Read the model definition and answer for the solid it produces. Units are mm, in the model's axes. Face numbers are marked on the shaded views. Round coordinates to 2 decimals unless told otherwise and drop trailing zeros. Write each loop counter-clockwise with the first axis right and the second up, starting at its lowest first coordinate (ties: lowest second). Pieces come first, ordered by that corner, then holes. Notation, with made-up numbers: (33.5, 85.5) -> (71.5, 85.5) arc R30 ccw to (71.5, 123.5) -> close; hole circle Ø3 at (-27.5, -33). An arc over 180 degrees is marked (long way). Return JSON: item names as keys, results as strings.
from build123d import *

# Parameters (mm, degrees)
SKETCH2_R           = 28.194
SKETCH2_R_2         = 25.654
BOSS_EXTRUDE1_DEPTH = 76.2
SKETCH3_R           = 9.652
CUT_EXTRUDE1_DEPTH  = 76.2
CIRPATTERN1_COUNT   = 2
CIRPATTERN1_ANGLE   = 60
CIRPATTERN2_COUNT   = 2
CIRPATTERN3_COUNT   = 2
CIRPATTERN3_ANGLE   = 120


with BuildPart() as part:
    # Sketch2 → Boss-Extrude1 (new body)
    with BuildSketch(Plane(origin=(0, 0, 0), x_dir=(1, 0, 0), z_dir=(0, 1, 0))):
        with Locations(Location((0, 0, 0), (0, 0, 90))):
            Circle(SKETCH2_R)
        with Locations(Location((0, 0, 0), (0, 0, 90))):
            Circle(SKETCH2_R_2, mode=Mode.SUBTRACT)
    extrude(amount=BOSS_EXTRUDE1_DEPTH)

    # Sketch3 → Cut-Extrude1 (cut)
    with BuildSketch(Plane.XY):
        with Locations(Location((0, 38.1, 0), (0, 0, 90))):
            Circle(SKETCH3_R)
    cut_extrude1 = extrude(amount=-CUT_EXTRUDE1_DEPTH, mode=Mode.SUBTRACT)

    # CirPattern1: Cut-Extrude1 ×2 about axis
    cirpattern1_axis = Axis((0, 76.2, 0), (0, -1, 0))
    for i in range(1, CIRPATTERN1_COUNT):
        add(cut_extrude1.rotate(cirpattern1_axis, i * CIRPATTERN1_ANGLE / (CIRPATTERN1_COUNT - 1)), mode=Mode.SUBTRACT)

    # CirPattern2: Cut-Extrude1 ×2 about axis
    cirpattern2_axis = Axis((0, 76.2, 0), (0, -1, 0))
    for i in range(1, CIRPATTERN2_COUNT):
        add(cut_extrude1.rotate(cirpattern2_axis, i * 360 / CIRPATTERN2_COUNT), mode=Mode.SUBTRACT)

    # CirPattern3: Cut-Extrude1 ×2 about axis
    cirpattern3_axis = Axis((0, 76.2, 0), (0, 1, 0))
    for i in range(1, CIRPATTERN3_COUNT):
        add(cut_extrude1.rotate(cirpattern3_axis, i * CIRPATTERN3_ANGLE / (CIRPATTERN3_COUNT - 1)), mode=Mode.SUBTRACT)


solid = part.part
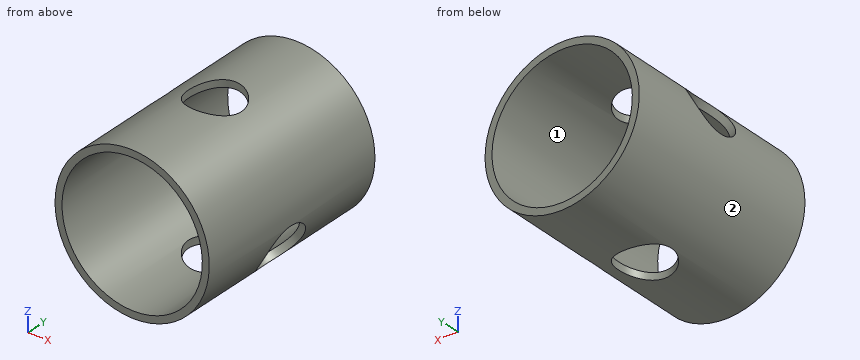
Item 1: Straight lines are drawn through the part: L1, parallel to X at y = 60, z = 0; L2, parallel to X at y = 52, z = 9; L3, parallel to Z at x = -14, y = 49. For each, find the intervals that lie inside material, in ascending order. Write a range as [from, to].
Worked answers:
{"L1": "x = [-28.19, -25.65], [25.65, 28.19]", "L2": "x = [-26.72, -24.02], [24.02, 26.72]", "L3": "z = [-24.47, -21.5], [21.5, 24.47]"}
Item 2: For a pull along X with two mould halves and no side action, classify the marked faces 1 and 2 as released by +X, released by -X, zero draft, split by the parting line, or undercut.
Worked answers:
{"face 1": "undercut", "face 2": "split by the parting line"}
Item 3: Flat-ended cylindrical pins translate along their axes: pin 1 (10 mm diameter, centred on x = -10, z = 20.5, fed in from +Y); pin 2 (4 mm diameter, centred on x = 20, y = 16.5, fed in from +Z); pin 3 (6 mm diameter, centred on x = -13.5, y = 21, fed in from +Z); pin 4 (4 mm diameter, centred on x = 8.5, y = 68, fed in from -Z). Find the tip coordinate at first contact, or state that the pin passes through.
Worked answers:
{"pin 1": "stops at y = 76.2", "pin 2": "stops at z = 21.7", "pin 3": "stops at z = 26.17", "pin 4": "stops at z = -27.43"}
Item 4: Section A-A (z = 0) is taken. Give the vertices of the cut face in (x, y), then the cut area to 3 significant figures.
Worked answers:
{"outline": "(-28.19, 0) -> (-25.65, 0) -> (-25.65, 76.2) -> (-28.19, 76.2) -> close; (25.65, 0) -> (28.19, 0) -> (28.19, 76.2) -> (25.65, 76.2) -> close", "area": "387 mm2"}
Item 5: Section B-B (x = 0) is taken. Give the vertices of the cut face in (y, z).
Worked answers:
{"outline": "(0, -28.19) -> (28.45, -28.19) -> (28.45, -25.65) -> (0, -25.65) -> close; (0, 25.65) -> (28.45, 25.65) -> (28.45, 28.19) -> (0, 28.19) -> close; (47.75, -28.19) -> (76.2, -28.19) -> (76.2, -25.65) -> (47.75, -25.65) -> close; (47.75, 25.65) -> (76.2, 25.65) -> (76.2, 28.19) -> (47.75, 28.19) -> close"}
Item 6: Section C-C (y = 38.1) is taken. Give the vertices of the cut face in (x, z).
Worked answers:
{"outline": "(-27.77, 4.89) arc R28.19 ccw to (-9.65, -26.49) -> (-9.65, -23.77) arc R25.65 cw to (-25.41, 3.53) -> close; (-18.12, 21.6) -> (-15.76, 20.24) arc R25.65 cw to (-9.65, 23.77) -> (-9.65, 26.49) arc R28.19 ccw to start; (9.65, -26.49) arc R28.19 ccw to (18.12, -21.6) -> (15.76, -20.24) arc R25.65 cw to (9.65, -23.77) -> close; (9.65, 23.77) arc R25.65 cw to (25.41, -3.53) -> (27.77, -4.89) arc R28.19 ccw to (9.65, 26.49) -> close"}
Item 7: Section D-D (x = 14.5) is taken. Give the vertices of the cut face in (y, z), then the cut area to 3 significant figures.
Worked answers:
{"outline": "(0, -24.18) -> (76.2, -24.18) -> (76.2, -21.16) -> (0, -21.16) -> close; (0, 21.16) -> (76.2, 21.16) -> (76.2, 24.18) -> (0, 24.18) -> close", "area": "460 mm2"}
